Study the drawing (mm; zero at the part's minimum x, y, z) and answer. A direction names the side the tool comes from. Give positions to 0.01 mm unless a question says otherwise; leave off trailing zeros. Loops run counter-clockwise (first coordinate to the right, second up) from the corner with the lowest first, then second, coordinate; pieces in that order, holes last. Notation, with made-up numbers: M 53,75.25 L 74,75.25 A28 ccw 74,113.25 Z; hole C -10.5,25 d1. An arc over 180 degrees is marked long. Use one line per item in the form item = value. Start each with the question number.
1. The mould has two halves that part along Z. Classify the marked faces 3, 4 and 5: released by +Z, released by -Z, zero draft, split by the parting line, or undercut.
2. The part is cut by section D-D (y = 11.5). Write down the section's boundary in (x, z).
3. Straight lines are drawn through the part: line 1 (Z direction, x = 10, y = 8.25); line 2 (X direction, y = 6, z = 8.25); line 3 (Y direction, x = 7.75, z = 1.5). For each, find the intervals that lie inside material, in ascending order. Write a range as from..to.
4. The part is cut by section A-A (x = 10). Write down the section's boundary in (y, z), and give its area (3 significant figures).
5. The part is cut by section B-B (z = 10). Write down the section's boundary in (x, y), and give its area (3 significant figures).
6. For the marked faces 1 and 2, determine the directions among +Z, -Z, +X, -X, +Y, -Y from which every point of the face is accessible in a straight line to the end or side of a thin tool.
7. The part is cut by section C-C (y = 2.25). Write down the section's boundary in (x, z).
8. Each of these flat-tipped pins is pushed along its axis until it touches: pin 1 Ø9.5 at (x, z) = (10, 10) entering from -Y; pin 2 Ø6 at (y, z) = (8.5, 4.5) entering from -X; pin 3 Ø4 at (y, z) = (6, 9.5) entering from -X; pin 4 Ø3 at (x, y) = (14.5, 11.5) entering from +Z. Where does it stop, or does it pass through?
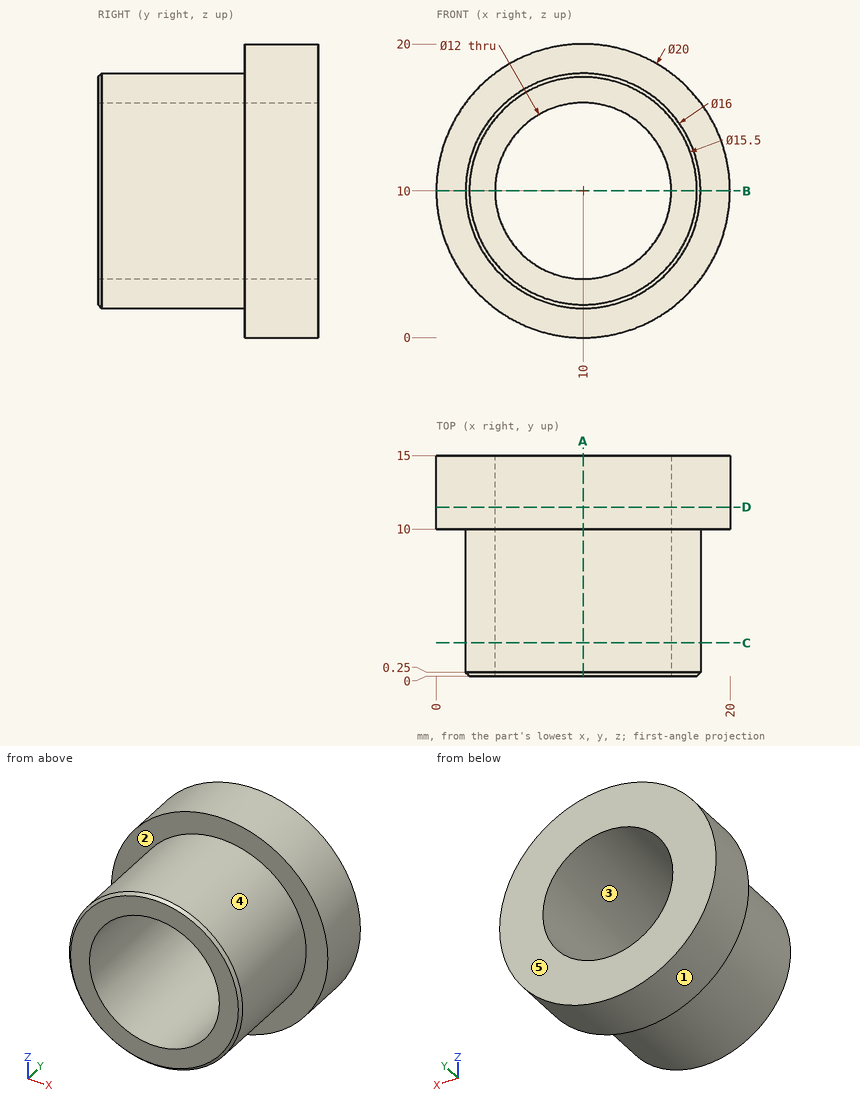
Derived:
q1.face_3 = undercut
q1.face_4 = split by the parting line
q1.face_5 = zero draft
q2.outline = C 10,10 d20; hole C 10,10 d12
q3.line_1 = 2..4, 16..18
q3.line_2 = 2.19..4.26, 15.74..17.81
q3.line_3 = 10..15
q4.outline = M 0,2.25 L 0.25,2 L 10,2 L 10,0 L 15,0 L 15,4 L 0,4 Z; M 0,16 L 15,16 L 15,20 L 10,20 L 10,18 L 0.25,18 L 0,17.75 Z
q4.area = 79.9 mm2
q5.outline = M 0,10 L 2,10 L 2,0.25 L 2.25,0 L 4,0 L 4,15 L 0,15 Z; M 16,0 L 17.75,0 L 18,0.25 L 18,10 L 20,10 L 20,15 L 16,15 Z
q5.area = 79.9 mm2
q6.face_1 = +Y, -Y
q6.face_2 = -Y
q7.outline = C 10,10 d16; hole C 10,10 d12
q8.pin_1 = through
q8.pin_2 = 0.43
q8.pin_3 = 2
q8.pin_4 = 19.54
